```python
from build123d import *

# Parameters (mm, degrees)
SKETCH1_W                      = 30
SKETCH1_H                      = 35
BASE_FLANGE1_DEPTH             = 2
EDGE_FLANGE1_STRIP_W           = 10
EDGE_FLANGE1_STRIP_H           = 2
EDGE_FLANGE1_STRIP_CUT_DEPTH   = 15
EDGE_FLANGE1_RELIEF_W          = 11
EDGE_FLANGE1_RELIEF_H          = 1
EDGE_FLANGE1_RELIEF_CUT_DEPTH  = 2
EDGE_FLANGE1_DEPTH             = 15
CUT_EXTRUDE1_REACH             = 1222.389
CUT_EXTRUDE2_REACH             = 1222.389
EDGE_FLANGE3_STRIP_CUT_DEPTH   = 37
EDGE_FLANGE3_STRIP_CUT_2_DEPTH = 37
EDGE_FLANGE3_DEPTH             = 37
EDGE_FLANGE3_BEND_DEPTH        = 37
FILLET5_R                      = 2


# Sheet-metal steps are written as plain solids
with BuildPart() as part:
    # Sketch1 → Base-Flange1 (new body)
    with BuildSketch(Plane(origin=(23.590386714, 0, 0), x_dir=(0, 0, -1), z_dir=(1, 0, 0))):
        with Locations((0.307827961, 1202.201275355)):
            Rectangle(SKETCH1_W, SKETCH1_H)
    extrude(amount=BASE_FLANGE1_DEPTH)

    # Edge-Flange1 strip (across the edge) → Edge-Flange1 strip cut (cut)
    with BuildSketch(Plane(origin=(25.590386714, 1184.701275355, 7.192172039), x_dir=(0, 1, 0), z_dir=(0, 0, -1))):
        with Locations((-4, -1)):
            Rectangle(EDGE_FLANGE1_STRIP_W, EDGE_FLANGE1_STRIP_H)
    extrude(amount=EDGE_FLANGE1_STRIP_CUT_DEPTH, mode=Mode.SUBTRACT)

    # Edge-Flange1 relief (on the sheet) → Edge-Flange1 relief cut (cut)
    with BuildSketch(Plane(origin=(25.590386714, 1185.701275355, 7.192172039), x_dir=(0, 1, 0), z_dir=(1, 0, 0))):
        with Locations((-4.5, 0.5)):
            Rectangle(EDGE_FLANGE1_RELIEF_W, EDGE_FLANGE1_RELIEF_H)
        with Locations((-4.5, -15.5)):
            Rectangle(EDGE_FLANGE1_RELIEF_W, EDGE_FLANGE1_RELIEF_H)
    extrude(amount=-EDGE_FLANGE1_RELIEF_CUT_DEPTH, mode=Mode.SUBTRACT)

    # Edge-Flange1 section (across the edge) → Edge-Flange1 (add)
    with BuildSketch(Plane(origin=(25.590386714, 1184.701275355, 7.192172039), x_dir=(0, 1, 0), z_dir=(0, 0, -1))):
        with BuildLine():
            Line((-2, 1), (-2, 38))
            Line((-2, 38), (0, 38))
            Line((0, 38), (0, 1))
            ThreePointArc((0, 1), (0.292893219, 0.292893219), (1, 0))
            Line((1, 0), (1, -2))
            ThreePointArc((1, -2), (-1.121320344, -1.121320344), (-2, 1))
        make_face()
    extrude(amount=EDGE_FLANGE1_DEPTH)

    # Sketch7 → Cut-Extrude1 (cut, up to next)
    with BuildSketch(Plane(origin=(25.590386714, 0, 0), x_dir=(0, 0, -1), z_dir=(1, 0, 0)), mode=Mode.PRIVATE) as cut_extrude1_sk1:
        with BuildLine():
            Line((-10.192172039, 1216.701275355), (-10.192172039, 1213.701275355))
            ThreePointArc((-10.192172039, 1213.701275355), (-11.692172039, 1212.201275355), (-13.192172039, 1213.701275355))
            Line((-13.192172039, 1213.701275355), (-13.192172039, 1216.701275355))
            ThreePointArc((-13.192172039, 1216.701275355), (-11.692172039, 1218.201275355), (-10.192172039, 1216.701275355))
        make_face()
    cut_extrude1_tool1 = extrude(cut_extrude1_sk1.sketch, amount=-CUT_EXTRUDE1_REACH, mode=Mode.PRIVATE) & part.part
    # Sketch7 → Cut-Extrude1 (cut, up to next)
    with BuildSketch(Plane(origin=(25.590386714, 0, 0), x_dir=(0, 0, -1), z_dir=(1, 0, 0)), mode=Mode.PRIVATE) as cut_extrude1_sk2:
        with BuildLine():
            Line((10.807827961, 1216.701275355), (10.807827961, 1213.701275355))
            ThreePointArc((10.807827961, 1213.701275355), (12.307827961, 1212.201275355), (13.807827961, 1213.701275355))
            Line((13.807827961, 1213.701275355), (13.807827961, 1216.701275355))
            ThreePointArc((13.807827961, 1216.701275355), (12.307827961, 1218.201275355), (10.807827961, 1216.701275355))
        make_face()
    cut_extrude1_tool2 = extrude(cut_extrude1_sk2.sketch, amount=-CUT_EXTRUDE1_REACH, mode=Mode.PRIVATE) & part.part
    add(cut_extrude1_tool1.solids().sort_by_distance((25.590387, 1215.201275, 11.692172))[0], mode=Mode.SUBTRACT)
    add(cut_extrude1_tool2.solids().sort_by_distance((25.590387, 1215.201275, -12.307828))[0], mode=Mode.SUBTRACT)

    # Sketch8 → Cut-Extrude2 (cut, up to next)
    with BuildSketch(Plane(origin=(25.590386714, 0, 0), x_dir=(0, 0, -1), z_dir=(1, 0, 0)), mode=Mode.PRIVATE) as cut_extrude2_sk1:
        with BuildLine():
            Line((-7.192172039, 1199.701275355), (-7.192172039, 1202.701275355))
            ThreePointArc((-7.192172039, 1202.701275355), (0.307827961, 1210.201275355), (7.807827961, 1202.701275355))
            Line((7.807827961, 1202.701275355), (7.807827961, 1199.701275355))
            ThreePointArc((7.807827961, 1199.701275355), (0.307827961, 1192.201275355), (-7.192172039, 1199.701275355))
        make_face()
    cut_extrude2_tool1 = extrude(cut_extrude2_sk1.sketch, amount=-CUT_EXTRUDE2_REACH, mode=Mode.PRIVATE) & part.part
    add(cut_extrude2_tool1.solids().sort_by_distance((25.590387, 1201.201275, -0.307828))[0], mode=Mode.SUBTRACT)

    # Edge-Flange3 strip (across the edge) → Edge-Flange3 strip cut (cut)
    with BuildSketch(Plane(origin=(26.590386714, 1184.701275355, 7.192172039), x_dir=(3.000602769257188e-15, 0.5000000000000041, -0.8660254037844364), z_dir=(1, 0, 0))):
        Polygon((-9.160254038, 2.979274058), (-0.5, -2.020725942), (0.5, -0.288675135), (-8.160254038, 4.711324865), align=None)
    extrude(amount=EDGE_FLANGE3_STRIP_CUT_DEPTH, mode=Mode.SUBTRACT)

    # Edge-Flange3 strip 2 (across the edge) → Edge-Flange3 strip cut 2 (cut)
    with BuildSketch(Plane(origin=(63.590386714, 1184.701275355, -7.807827961), x_dir=(2.9396981233624387e-15, 0.5000000000000041, 0.8660254037844364), z_dir=(-1, 0, 0))):
        Polygon((-9.160254038, 2.979274058), (-0.5, -2.020725942), (0.5, -0.288675135), (-8.160254038, 4.711324865), align=None)
    extrude(amount=EDGE_FLANGE3_STRIP_CUT_2_DEPTH, mode=Mode.SUBTRACT)

    # Edge-Flange3 section (across the edge) → Edge-Flange3 (add)
    with BuildSketch(Plane(origin=(26.590386714, 1184.701275355, 7.192172039), x_dir=(3.000602769257188e-15, 0.5000000000000041, -0.8660254037844364), z_dir=(1, 0, 0))):
        with BuildLine():
            Line((-2, 0.577350269), (-2, 10.845299462))
            Line((-2, 10.845299462), (0, 10.845299462))
            Line((0, 10.845299462), (0, 0.577350269))
            ThreePointArc((0, 0.577350269), (0.133974596, 0.077350269), (0.5, -0.288675135))
            Line((0.5, -0.288675135), (-0.5, -2.020725942))
            ThreePointArc((-0.5, -2.020725942), (-1.598076211, -0.922649731), (-2, 0.577350269))
        make_face()
    extrude(amount=EDGE_FLANGE3_DEPTH)

    # Edge-Flange3 section 2 (across the edge) → Edge-Flange3 bend (add)
    with BuildSketch(Plane(origin=(63.590386714, 1184.701275355, -7.807827961), x_dir=(2.9396981233624387e-15, 0.5000000000000041, 0.8660254037844364), z_dir=(-1, 0, 0))):
        with BuildLine():
            Line((-2, 0.577350269), (-2, 10.845299462))
            Line((-2, 10.845299462), (0, 10.845299462))
            Line((0, 10.845299462), (0, 0.577350269))
            ThreePointArc((0, 0.577350269), (0.133974596, 0.077350269), (0.5, -0.288675135))
            Line((0.5, -0.288675135), (-0.5, -2.020725942))
            ThreePointArc((-0.5, -2.020725942), (-1.598076211, -0.922649731), (-2, 0.577350269))
        make_face()
    extrude(amount=EDGE_FLANGE3_BEND_DEPTH)

    # Fillet5
    fillet5_edges = [part.edges().sort_by_distance(p)[0] for p in [
        (63.590386714, 1193.5935802, 13.480847173),
        (63.590386714, 1193.5935802, -14.096503096),
        (24.590386714, 1219.701275355, 14.692172039),
        (24.590386714, 1219.701275355, -15.307827961),
    ]]
    fillet(fillet5_edges, radius=FILLET5_R)


solid = part.part
```
Work out the finished part from the listing and answer in its coordinate system (mm). A direction names the side the tool comes from. Coordinates: 2 decimals unless noted, no trailing zeros. Loops run counter-clockwise (first coordinate to the right, second up) from the corner with the lowest first, then second, coordinate; pieces in that order, holes last. Notation, with made-up numbers: M 70.25,53.5 L 122.25,53.5 A24 ccw 122.25,63.5 Z; hole C 84,-3 d8. An arc over 180 degrees is marked long. Use CSV: the item, a comma, the result in double quotes. Start each with the question number.
(1) Given pin 1 Ø12 at (x, y) = (59, 1197) entering from -Z; pin 2 Ø1.5 at (x, z) = (51.5, -10.5) entering from -Y; pin 3 Ø1.6 at (x, z) = (25, -13.5) entering from -Y, each flat-ended and moving along its own axis, determine where each tip first touches the part or whether it passes through.
(2) Find section C-C, the plane y = 1196.5. Give the vertices of the cut face in (x, z), then the cut area to 3 significant figures.
(3) For faces 4 (the face through (25, 1201, 7.192)), 5 (the face through (25, 1185, -7.808)), 6 (the face through (44.831, 1188.585, 11.744)), 7 (the face through (25, 1184.701, 11)), determine the directions among +Z, -Z, +X, -X, +Y, -Y from which every point of the face is accessible in a straight line to the end or side of a thin tool.
(4) Find section A-A, the plane x = 31. Give the vertices of the cut face in (y, z).
(5) For a pull along Z with two mould halves and no side action, classify faces 1 (the face through (45, 1182.701, 0)), 2 (the face through (25, 1215, 10.192)), 3 (the face through (24.6, 1219.13, -14.71)) as +Z half, -Z half, draft (parallel to the pull), parting line (faces both ways), or undercut.
(6) Find section D-D, the plane y = 1213. Give the vertices of the cut face in (x, z).
(7) Find section B-B, the plane z = 0.75. Give the vertices of the cut face in (x, y), then the cut area to 3 significant figures.
(8) Consider line 1 (X direction, y = 1211.5, z = -7.75); line 2 (Y direction, x = 50.5, z = 6.25); line 3 (Z direction, x = 48, y = 1191.5). Determine where each line is inside the solid, lowest interval first.
Recorded:
1,pin 1,"stops at z = -14.96"
1,pin 2,"stops at y = 1184.07"
1,pin 3,"stops at y = 1184.7"
2,outline,"M 23.59,-15.31 L 25.59,-15.31 L 25.59,-7.09 L 23.59,-7.09 Z; M 23.59,6.47 L 25.59,6.47 L 25.59,14.69 L 23.59,14.69 Z"
2,area,"32.9 mm^2"
3,face 4,"+X, -X"
3,face 5,"-X, -Y"
3,face 6,"+Z, +X, -Y"
3,face 7,"+Z, -X, -Y"
4,outline,"M 1182.7,-7.23 A3 ccw 1184.2,-9.83 L 1193.09,-14.96 L 1194.09,-13.23 L 1185.2,-8.1 A1 cw 1184.7,-7.23 L 1184.7,6.61 A1 cw 1185.2,7.48 L 1194.09,12.61 L 1193.09,14.35 L 1184.2,9.21 A3 ccw 1182.7,6.61 Z"
5,face 1,"draft"
5,face 2,"undercut"
5,face 3,"-Z half"
6,outline,"M 23.59,-15.31 L 25.59,-15.31 L 25.59,-13.63 L 23.59,-13.63 Z; M 23.59,-10.98 L 25.59,-10.98 L 25.59,10.37 L 23.59,10.37 Z; M 23.59,13.02 L 25.59,13.02 L 25.59,14.69 L 23.59,14.69 Z"
7,outline,"M 23.59,1185.7 A3 ccw 26.59,1182.7 L 63.59,1182.7 L 63.59,1184.7 L 26.59,1184.7 A1 cw 25.59,1185.7 L 25.59,1192.28 L 23.59,1192.28 Z; M 23.59,1210.13 L 25.59,1210.13 L 25.59,1219.7 L 23.59,1219.7 Z"
7,area,"113 mm^2"
8,line 1,"x = 23.59 to 25.59"
8,line 2,"y = 1182.7 to 1184.7"
8,line 3,"z = -14.04 to -11.73, 11.12 to 13.43"
